Geometry check sheet. Reference: drawing and pictorial views, mm from the part's lowest x, y, z. Round coordinates to 2 decimals unless told otherwise and drop trailing zeros. Order: outer loops, then holes, each group sorted by start corner. A loop starts at its lowest first (then second) coordinate and runs counter-clockwise, first axis right, second up.
(1) Cross-section at D-D on x = 10.75. Enter the section's corners in (y, z).
(2) Thickness scan on L1, parallel to X at y = 8, z = 19; L2, parallel to Z at x = 8.75, y = 6.5; L3, parallel to Z at x = 3.5, y = 16.5 (1 decimal). Record the ranges inside material, lowest first.
(3) Cross-section at C-C on x = 3.5. Enter the section's corners in (y, z).
(4) Draft check along Y on the marked faces 1, 2 and 3. Enter one of: pulls with the +Y half, pulls with the -Y half, needs draft (parallel to the pull), parting line crosses it, or undercut.
(5) Gauge pin test, flat ends, axial feed: P1, Ø4, axis at x = 10.5, y = 9.5, coming from the +Z side; P2, Ø1.5, axis at y = 14.5, z = 24.5, coming from the -X side; P3, Ø2, axis at x = 4.5, z = 4.5, coming from the +Y side; P4, Ø12, axis at x = 13.5, z = 7, coming from the -Y side. Record the tip position at first contact, or that the pin passes through.
(6) Cross-section at A-A on z = 17.25. Enter the section's corners in (x, y).
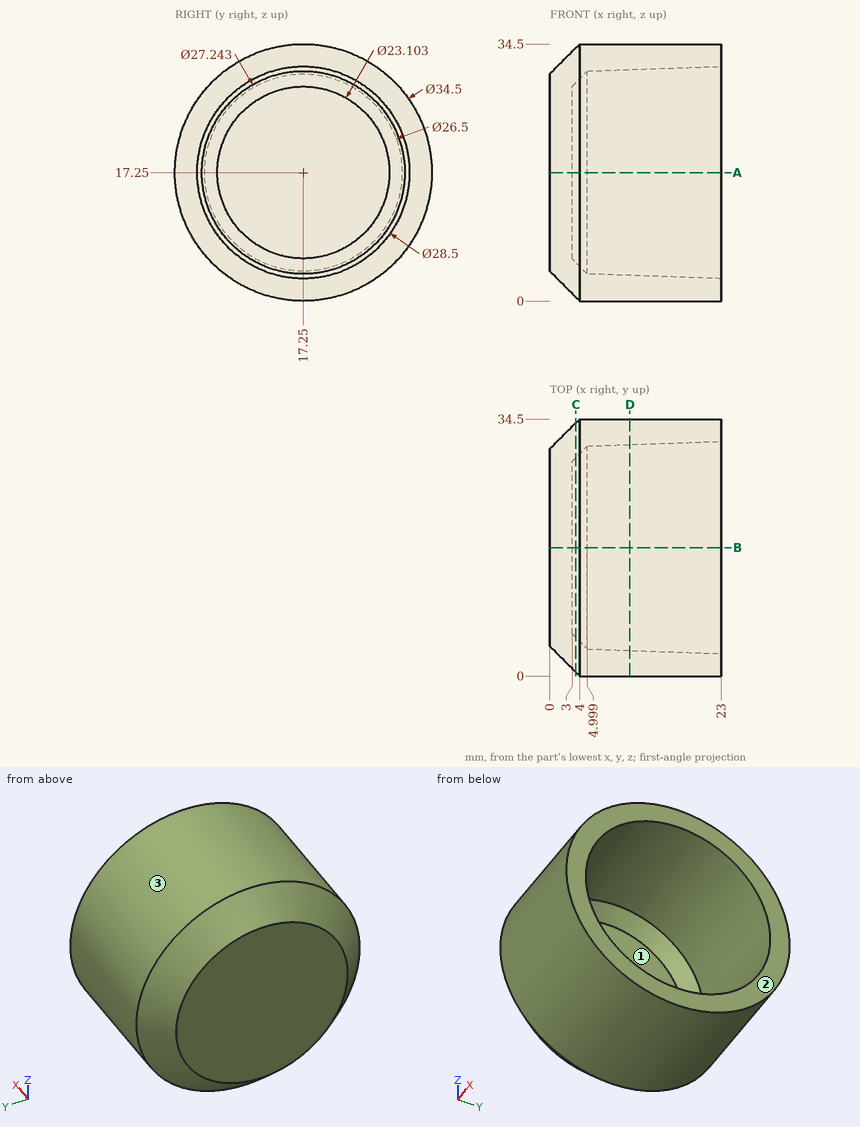
Found:
1. outline: circle Ø34.5 at (17.25, 17.25); hole circle Ø27.64 at (17.25, 17.25)
2. L1: x = 0 to 3
2. L2: z = 3.76 to 8.67, 25.83 to 30.74
2. L3: z = 0.5 to 5.2, 29.3 to 34
3. outline: circle Ø33.5 at (17.25, 17.25); hole circle Ø24.14 at (17.25, 17.25)
4. face 1: undercut
4. face 2: needs draft
4. face 3: parting line crosses it
5. P1: stops at z = 33.51
5. P2: stops at x = 0
5. P3: stops at y = 29.88
5. P4: stops at y = 0.53
6. outline: (0, 4) - (4, 0) - (23, 0) - (23, 3) - (5, 3.63) - (3, 5.7) - (3, 28.8) - (5, 30.87) - (23, 31.5) - (23, 34.5) - (4, 34.5) - (0, 30.5) - close
